Build history of the part. All positions in model axes, mm. A direction names the side the tool comes from. Coordinates: 2 decimals unless noted, no trailing zeros. Order: outer loops, then holes, each group sorted by start corner. A loop starts at its lowest first (then second) coordinate and runs counter-clockwise, first axis right, second up. Notation, with made-up numbers: (47, 33) - (52, 33) arc R20 cw to (52, 64) - close; hole circle Ø10 at (35, 24.25). An arc over 180 degrees is marked (long way). Write each question's results on one line, items separated by ' | '.
from build123d import *

# Parameters (mm, degrees)
F0_W      = 60
F0_H      = 110
F1_DEPTH  = 6.7
F2_W      = 56
F2_H      = 105
F3_DEPTH  = 5.1
F5_DEPTH  = 5.1
F6_R      = 3
F7_R      = 6
F9_DEPTH  = 19
F10_W     = 2
F10_H     = 19
F11_DEPTH = 4
F13_DEPTH = 25


with BuildPart() as f1:
    # F0 (on Top) → F1 (new body)
    with BuildSketch(Plane.XY):
        Rectangle(F0_W, F0_H)
    extrude(amount=F1_DEPTH)

    # F2 (on face) → F3 (cut)
    with BuildSketch(Plane.XY.offset(6.7)):
        with Locations((0, 2.5)):
            Rectangle(F2_W, F2_H)
    extrude(amount=-F3_DEPTH, mode=Mode.SUBTRACT)

    # F4 (on face) → F5 (join)
    with BuildSketch(Plane.XY.offset(1.6)):
        with BuildLine():
            Line((-28, -2.277589744), (-28, -5))
            ThreePointArc((-28, -5), (-24.8064638622, 22.5), (-28, 50))
            Line((-28, 50), (-28, 47.6836016319))
            ThreePointArc((-28, 47.6836016319), (-25.3710775237, 22.703005944), (-28, -2.277589744))
        make_face()
        with BuildLine():
            Line((28, 47.3302031996), (28, 50))
            ThreePointArc((28, 50), (24.8064638622, 22.5), (28, -5))
            Line((28, -5), (28, -2.2991948615))
            ThreePointArc((28, -2.2991948615), (25.4062635127, 22.515504169), (28, 47.3302031996))
        make_face()
    extrude(amount=F5_DEPTH)

    # F6
    f6_edges = [f1.edges().sort_by_distance(p)[0] for p in [
        (-30, -55, 3.35),
        (30, -55, 3.35),
    ]]
    fillet(f6_edges, radius=F6_R)

    # F7
    f7_edges = [f1.edges().sort_by_distance(p)[0] for p in [
        (28, -5, 4.15),
        (-28, -5, 4.15),
        (-28, 50, 4.15),
        (28, 50, 4.15),
    ]]
    fillet(f7_edges, radius=F7_R)

    # F8 (on face) → F9 (join)
    with BuildSketch(Plane(origin=(0, -50, 0), x_dir=(-1, 0, 0), z_dir=(0, 1, 0))):
        Polygon((-15.25, 2.4), (-23, 1.6), (28, 1.6), (28, 4.8), (23, 4.8), (15.25, 4), (10.25, 4), (2.5, 3.2), (-2.5, 3.2), (-10.25, 2.4), align=None)
    extrude(amount=F9_DEPTH)

    # F10 (on face) → F11 (cut)
    with BuildSketch(Plane.XY.offset(6.7)):
        with Locations((29, -40.5)):
            Rectangle(F10_W, F10_H)
    extrude(amount=-F11_DEPTH, mode=Mode.SUBTRACT)

    # F12 (on face) → F13 (cut)
    with BuildSketch(Plane(origin=(0, -50, 0), x_dir=(-1, 0, 0), z_dir=(0, 1, 0))):
        Polygon((23, 4.8), (28, 4.8), (28, 6.7), (-29.9160797831, 6.7), (-29.9160797831, 2.7), (-28, 2.7), (-28, 1.6), (-23, 1.6), (-15.25, 2.4), (-10.25, 2.4), (-2.5, 3.2), (2.5, 3.2), (10.25, 4), (15.25, 4), align=None)
    extrude(amount=-F13_DEPTH, mode=Mode.SUBTRACT)


solid = f1.part
1. Two-plate mould, pull along X, no slides. Class faces 5 (the face through (28, 22, 4)), 6 (the face through (30, 1, 3)), 7 (the face through (0, 1, 0)): +X half, -X half, draft (parallel to the pull), parting line (faces both ways), or undercut.
Solved:
face 5: undercut | face 6: +X half | face 7: draft
2. Tool access for faces 1 (the face through (6.321, -43.168, 2.806)), 2 (the face through (-28, 53, 4)), 3 (the face through (-28, 22, 4)), 4 (the face through (-29.14, -54.1, 3.4)): list every direction of +Z, -Z, +X, -X, +Y, -Y with a clear straight run to the whole face (end or side of a thin tool).
Solved:
face 1: +Z, +Y, -Y | face 2: +Z, +Y | face 3: +Z | face 4: +Z, -Z, -X, -Y
3. Band-saw the part on D-D on x = 19. Give the cut face in (y, z), then the cut area to 3 significant figures.
Solved:
outline: (-55, 0) - (55, 0) - (55, 1.6) - (-31, 1.6) - (-31, 2.01) - (-55, 2.01) - close | area: 186 mm2
4. Drop flat-ended pins along their axis: pin 1 Ø8 at (x, y) = (-16.5, 18.5) entering from +Z; pin 2 Ø1.5 at (x, y) = (1, -39) entering from +Z; pin 3 Ø2 at (x, z) = (2.5, 6) entering from +Y; pin 4 Ø2 at (x, z) = (29.5, 5.5) entering from -Y. Give the stop position or say it passes through.
Solved:
pin 1: stops at z = 1.6 | pin 2: stops at z = 3.2 | pin 3: passes through | pin 4: stops at y = -52.7
5. Probe line 1 (X direction, y = 23, z = 2.25); line 2 (X direction, y = 37.5, z = 6.25); line 3 (X direction, y = -10.5, z = 1.75). List the from-to ranges inside material, lowest first.
Solved:
line 1: x = -30 to -28, -25.37 to -24.81, 24.81 to 25.41, 28 to 30 | line 2: x = -30 to -28, -26.29 to -25.75, 25.75 to 26.35, 28 to 30 | line 3: x = -30 to -28, 28 to 30
6. Band-saw the part on C-C on y = -12. Give the cut face in (x, z).
Solved:
outline: (-30, 0) - (30, 0) - (30, 6.7) - (28, 6.7) - (28, 1.6) - (-28, 1.6) - (-28, 6.7) - (-30, 6.7) - close
7. Band-saw the part on B-B on x = -12. Give the cut face in (y, z), then the cut area to 3 significant figures.
Solved:
outline: (-55, 0) - (55, 0) - (55, 1.6) - (-31, 1.6) - (-31, 4) - (-55, 4) - close | area: 234 mm2
8. Band-saw the part on A-A on y = -37.5. Give the cut face in (x, z), then the cut area to 3 significant figures.
Solved:
outline: (-30, 0) - (30, 0) - (30, 2.7) - (28, 2.7) - (28, 1.6) - (23, 1.6) - (15.25, 2.4) - (10.25, 2.4) - (2.5, 3.2) - (-2.5, 3.2) - (-10.25, 4) - (-15.25, 4) - (-23, 4.8) - (-28, 4.8) - (-28, 6.7) - (-30, 6.7) - close | area: 198 mm2
